```python
from build123d import *

# Parameters (mm, degrees)
SKETCH1_R           = 3.5
BOSS_EXTRUDE1_DEPTH = 1.651
BOSS_EXTRUDE2_DEPTH = 0.508
FILLET1_R           = 0.254
SKETCH3_W           = 4.699
SKETCH3_H           = 6.096
BOSS_EXTRUDE3_DEPTH = 1.016


with BuildPart() as part:
    # Sketch1 → Boss-Extrude1 (new body)
    with BuildSketch(Plane(origin=(0, 0, 0), x_dir=(1, 0, 0), z_dir=(0, 1, 0))):
        Polygon((0, 85.598), (0, 0), (14.605, 0), (14.605, 93.726), (1.143, 93.726), (1.143, 85.598), align=None)
        with Locations((7, 44.3)):
            Circle(SKETCH1_R, mode=Mode.SUBTRACT)
    extrude(amount=BOSS_EXTRUDE1_DEPTH)

    # Sketch2 → Boss-Extrude2 (add)
    with BuildSketch(Plane(origin=(0, 1.651, 0), x_dir=(1, 0, 0), z_dir=(0, 1, 0))):
        with BuildLine():
            Line((1.778, 3.556), (10.668, 3.556))
            ThreePointArc((10.668, 3.556), (12.446, 1.778), (10.668, 0))
            Line((10.668, 0), (1.778, 0))
            ThreePointArc((1.778, 0), (0, 1.778), (1.778, 3.556))
        make_face()
    extrude(amount=BOSS_EXTRUDE2_DEPTH)

    # Fillet1
    fillet1_edges = [part.edges().sort_by_distance(p)[0] for p in [
        (6.223, 2.159, -3.556),
        (6.223, 2.159, 0),
        (12.446, 2.159, -1.778),
        (0, 2.159, -1.778),
    ]]
    fillet(fillet1_edges, radius=FILLET1_R)

    # Sketch3 → Boss-Extrude3 (add)
    with BuildSketch(Plane.XZ):
        with Locations((12.2555, -8.763)):
            Rectangle(SKETCH3_W, SKETCH3_H)
        with Locations((12.2555, -22.225)):
            Rectangle(SKETCH3_W, SKETCH3_H)
        with Locations((12.2555, -56.896)):
            Rectangle(SKETCH3_W, SKETCH3_H)
        with Locations((12.2555, -70.485)):
            Rectangle(SKETCH3_W, SKETCH3_H)
        with Locations((2.3495, -75.946)):
            Rectangle(SKETCH3_W, SKETCH3_H)
        with Locations((2.3495, -62.357)):
            Rectangle(SKETCH3_W, SKETCH3_H)
        with Locations((2.3495, -27.686)):
            Rectangle(SKETCH3_W, SKETCH3_H)
        with Locations((2.3495, -14.224)):
            Rectangle(SKETCH3_W, SKETCH3_H)
    extrude(amount=BOSS_EXTRUDE3_DEPTH)


solid = part.part
```
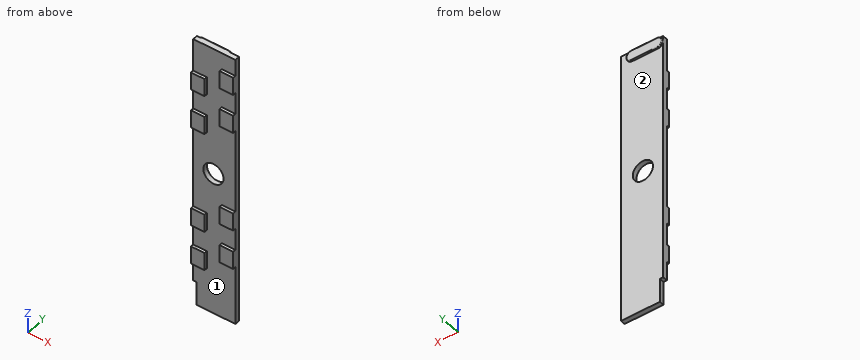
The model under review builds one solid part; all positions refer to its coordinate system, in mm. Face numbers are marked on the shaded views. Give positions to 0.01 mm unless a question says otherwise; leave off trailing zeros. Order: outer loops, then holes, each group sorted by start corner. A loop starts at its lowest first (then second) coordinate and runs counter-clockwise, first axis right, second up. Notation, with made-up numbers: (32.25, -18.75) - (62.25, -18.75) arc R18 cw to (62.25, -4.75) - close; hole circle Ø11 at (-30.5, 61.25). An arc over 180 degrees is marked (long way). Use CSV: the item, a comma, the result in double quotes. Start each with the question number.
Q1. Clearance check with flat-ended pins moving along their axes: pin 1 Ø0.8 at (x, y) = (13.5, -0.5) entering from +Z (3 decimals); pin 2 Ø5 at (x, z) = (8, -35) entering from +Y; pin 3 Ø5 at (x, z) = (4, -20) entering from -Y. State where each tip first meets the part, or that it passes through.
Q2. We need section D-D, the plane z = -13.5. Write out the cut boundary in (x, y) (3 decimals).
Q3. We need section B-B, the plane z = -44.3. Write out the cut boundary in (x, y) (3 decimals), and give its area (3 significant figures).
Q4. The part is to be moulded in two halves that separate along Z. For the marked faces 1 and 2, say which applies: +Z half, -Z half, draft (parallel to the pull), parting line (faces both ways), or undercut.
Q5. We need section C-C, the plane x = 7. Write out the cut boundary in (y, z) (3 decimals), and give its area (3 significant figures).
Q6. We need section A-A, the plane y = 1.1. Write out the cut boundary in (x, z) (3 decimals).
Q7. To check wall thickness, follow line 1 along Z through (x, y) = (7, 0.35); line 2 along X through (y, z) = (1.05, -44.3) (3 decimals); line 3 along Y through (x, z) = (1, -13). State the ranges of each line that lie inside material, in increasing order. Write a range as [from, to].
Outcome:
1,pin 1,"stops at z = -5.715"
1,pin 2,"stops at y = 1.65"
1,pin 3,"stops at y = 0"
2,outline,"(0, -1.016) - (4.699, -1.016) - (4.699, 0) - (14.605, 0) - (14.605, 1.651) - (0, 1.651) - close"
3,outline,"(0, 0) - (3.5, 0) - (3.5, 1.651) - (0, 1.651) - close; (10.5, 0) - (14.605, 0) - (14.605, 1.651) - (10.5, 1.651) - close"
3,area,"12.6 mm^2"
4,face 1,"undercut"
4,face 2,"draft"
5,outline,"(0, -93.726) - (1.651, -93.726) - (1.651, -47.8) - (0, -47.8) - close; (0, -40.8) - (1.651, -40.8) - (1.651, -3.556) - (1.905, -3.556) arc R0.254 ccw to (2.159, -3.302) - (2.159, -0.254) arc R0.254 ccw to (1.905, 0) - (0, 0) - close"
5,area,"145 mm^2"
6,outline,"(0, -85.598) - (1.143, -85.598) - (1.143, -93.726) - (14.605, -93.726) - (14.605, 0) - (0, 0) - close; hole circle Ø7 at (7, -44.3)"
7,line 1,"z = [-93.73, -47.8], [-40.8, 0]"
7,line 2,"x = [0, 3.5], [10.5, 14.605]"
7,line 3,"y = [-1.02, 1.65]"
